Here's how the part is built. I have some questions about the finished solid (model axes, mm). Coordinates: 2 decimals unless noted, no trailing zeros. Order: outer loops, then holes, each group sorted by start corner. A loop starts at its lowest first (then second) coordinate and runs counter-clockwise, first axis right, second up. Notation, with made-up numbers: (80, 25) - (91, 25) arc R23 cw to (91, 53) - close; hole circle Ø2 at (7.5, -4). An arc over 180 degrees is marked (long way). Answer as CSV lines item,"result". Start each with the question number.
Item 1: Imagine slicing it at A-A on y = 628. List the corners of the cut face in (x, z) for me, and give its area (3 significant figures).
Item 2: I need wall thicknesses on line 1 (Z direction, x = 0.25, y = 549); line 2 (Z direction, x = 1.8, y = 66); line 3 (Y direction, x = 0.45, z = 480). Which ranges of each line are inside material? Lowest first, please.
Item 3: Imagine slicing it at B-B on y = -142.5. List the corners of the cut face in (x, z) for me, and give its area (3 significant figures).
Item 4: I'm going to push flat-ended pins straight in: pin 1 (1 mm diameter, centred on x = 1, z = 498.5, fed in from +Y); pin 2 (0.8 mm diameter, centred on x = 1, y = 627, fed in from -Z); pin 3 (1 mm diameter, centred on x = 2, z = 806.5, fed in from -Y). Where does each tip first touch, or does it pass through?
from build123d import *

# Parameters (mm, degrees)
BOSS_EXTRUDE3_DEPTH = 2.54


with BuildPart() as part:
    # Sketch1 → Boss-Extrude3 (new body)
    with BuildSketch(Plane(origin=(0, 0, 0), x_dir=(0, 0, -1), z_dir=(1, 0, 0))):
        with BuildLine():
            Line((-328.770779224, -230.923937708), (-1.3867e-05, -230.923937708))
            Line((-1.3867e-05, -230.923937708), (-1.3866e-05, -78.523920986))
            add(Edge.make_bspline(
                [(-1.3866e-05, -78.523920986), (-663.575061276, -78.523963202), (-1327.150157835, 585.051089401)],
                knots=[0, 0, 0, 1, 1, 1], degree=2))
            Line((-1327.150157835, 585.051089401), (-1327.149864381, 694.252697447))
            ThreePointArc((-1327.149864381, 694.252697447), (-1330.869609261, 703.232955586), (-1339.849867516, 706.952700185))
            Line((-1339.849867516, 706.952700185), (-1432.872655994, 706.952698728))
            ThreePointArc((-1432.872655994, 706.952698728), (-1441.852912057, 703.232954709), (-1445.572655795, 694.25269853))
            Line((-1445.572655795, 694.25269853), (-1445.572655378, 667.601090483))
            ThreePointArc((-1445.572655378, 667.601090483), (-1441.852911359, 658.620834421), (-1432.872655179, 654.901090682))
            Line((-1432.872655179, 654.901090682), (-1401.368674128, 654.901091175))
            ThreePointArc((-1401.368674128, 654.901091175), (-1389.659272694, 666.610488308), (-1377.949874128, 654.901088308))
            Line((-1377.949874128, 654.901088308), (-1377.949874128, 534.251091161))
            Line((-1377.949874128, 534.251091161), (-880.381692198, 89.86268528))
            Line((-880.381692198, 89.86268528), (-328.770779224, -230.923937708))
        make_face()
    extrude(amount=BOSS_EXTRUDE3_DEPTH)


solid = part.part
Responses:
1,outline,"(0, 1327.15) - (2.54, 1327.15) - (2.54, 1377.95) - (0, 1377.95) - close"
1,area,"129 mm^2"
2,line 1,"z = 1290.6 to 1377.95"
2,line 2,"z = 619.36 to 839.35"
2,line 3,"y = -142.98 to 8.28"
3,outline,"(0, 0) - (2.54, 0) - (2.54, 480.82) - (0, 480.82) - close"
3,area,"1,220 mm^2"
4,pin 1,"stops at y = 15.29"
4,pin 2,"stops at z = 1327.15"
4,pin 3,"stops at y = 46.61"
